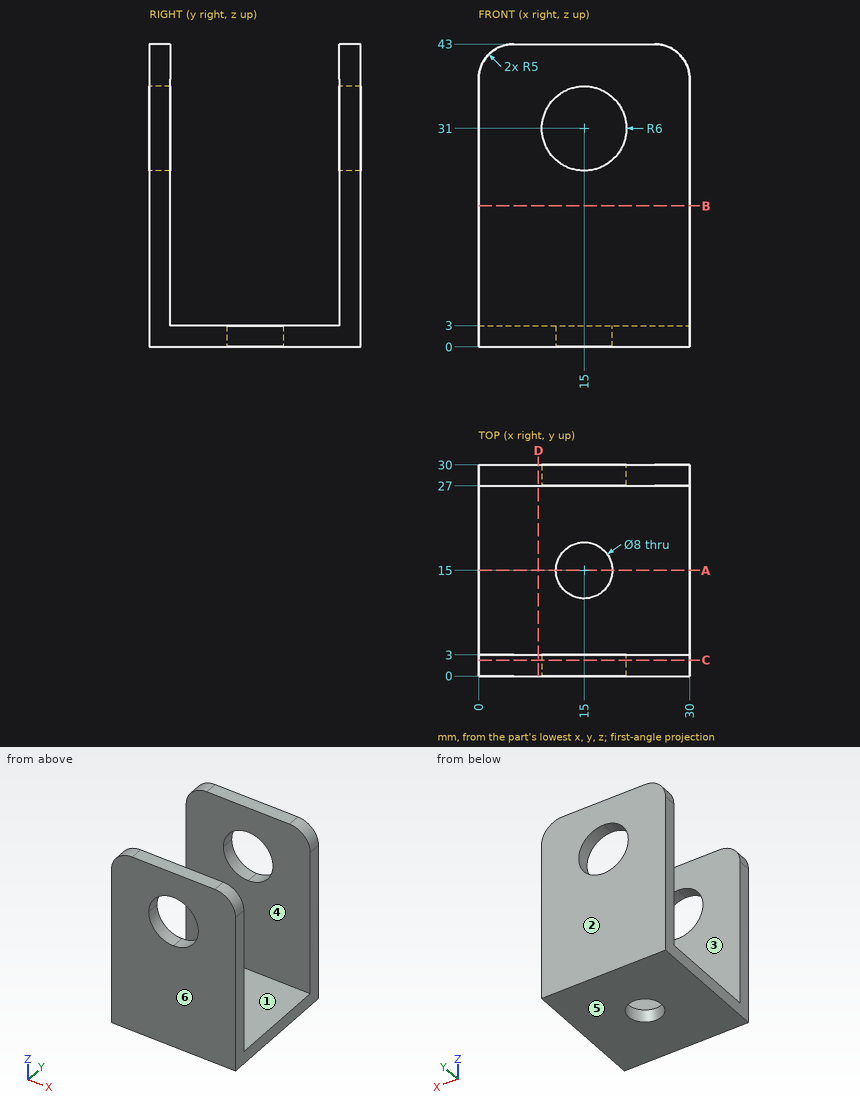
Can you work these out from the drawing? Everything is in mm from the part's minimum corner. A direction names the side the tool comes from. Round coordinates to 2 decimals unless told otherwise and drop trailing zeros. Write each loop counter-clockwise with the first axis right and the second up, starting at its lowest first coordinate (ties: lowest second). Pieces come first, ordered by that corner, then holes.
1. Suppose I cut it at A-A (y = 15). List the corners of the cut face in (x, z) for me.
2. If we mould it in two halves opening along Y, with no side actions, what happens to the marked faces 3, 4, 5 and 6? For each: released by +Y, released by -Y, zero draft, split by the parting line, or undercut.
3. Suppose I cut it at D-D (x = 8.5). List the corners of the cut face in (y, z) for me.
4. Suppose I cut it at C-C (y = 2.25). List the corners of the cut face in (x, z) for me.
5. Suppose I cut it at B-B (z = 20). List the corners of the cut face in (x, y) for me, and give its area (3 significant figures).
6. For the marked faces 1 and 2, which set-ups out of +Z, -Z, +X, -X, +Y, -Y let a thin tool reach every point of the face, with its end or its side?
7. I need wall thicknesses on L1, parallel to Y at x = 15, z = 1; L2, parallel to Y at x = 27.25, z = 32. Which ranges of each line are inside material? Lowest first, please.
8. Will these pins go through, and if not, where does the flat tip stop? pin 1 Ø2 at (x, z) = (5.5, 24) entering from -Y; pin 2 Ø12 at (x, y) = (14.5, 12) entering from +Z.
Answer sheet:
1. outline: (0, 0) - (11, 0) - (11, 3) - (0, 3) - close; (19, 0) - (30, 0) - (30, 3) - (19, 3) - close
2. face 3: undercut
2. face 4: undercut
2. face 5: zero draft
2. face 6: released by -Y
3. outline: (0, 0) - (30, 0) - (30, 43) - (27, 43) - (27, 3) - (3, 3) - (3, 43) - (0, 43) - close
4. outline: (0, 0) - (30, 0) - (30, 38) arc R5 ccw to (25, 43) - (5, 43) arc R5 ccw to (0, 38) - close; hole (9, 31) arc R6 ccw to (15, 25) arc R6 ccw to (15, 37) arc R6 ccw to start
5. outline: (0, 0) - (30, 0) - (30, 3) - (0, 3) - close; (0, 27) - (30, 27) - (30, 30) - (0, 30) - close
5. area: 180 mm2
6. face 1: +Z, +X, -X
6. face 2: +Z, -Z, +X, -X, +Y
7. L1: y = 0 to 11, 19 to 30
7. L2: y = 0 to 3, 27 to 30
8. pin 1: stops at y = 0
8. pin 2: stops at z = 3
